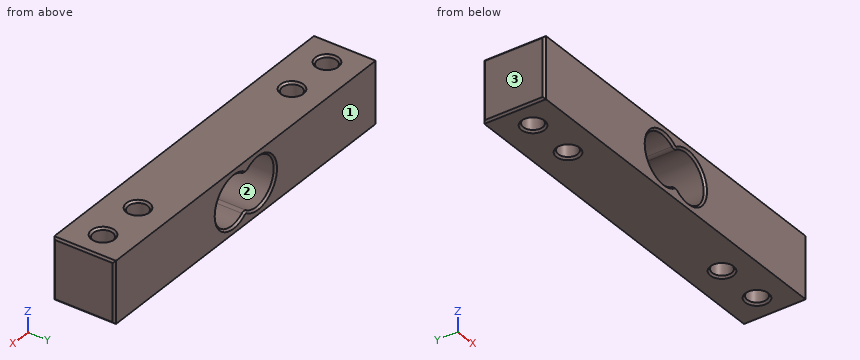
```python
from build123d import *

# Parameters (mm, degrees)
SKETCH1_W           = 75
SKETCH1_H           = 12.7
SKETCH1_R           = 2
BOSS_EXTRUDE1_DEPTH = 12.7
CUT_EXTRUDE1_REACH  = 14.7
FILLET1_R           = 1
CHAMFER1_SIZE       = 0.4


with BuildPart() as part:
    # Sketch1 → Boss-Extrude1 (new body)
    with BuildSketch(Plane.XY):
        Rectangle(SKETCH1_W, SKETCH1_H)
        with Locations((-32, 0)):
            Circle(SKETCH1_R, mode=Mode.SUBTRACT)
        with Locations((-22, 0)):
            Circle(SKETCH1_R, mode=Mode.SUBTRACT)
        with Locations((22, 0)):
            Circle(SKETCH1_R, mode=Mode.SUBTRACT)
        with Locations((32, 0)):
            Circle(SKETCH1_R, mode=Mode.SUBTRACT)
    extrude(amount=BOSS_EXTRUDE1_DEPTH)

    # Sketch2 → Cut-Extrude1 (cut, up to next)
    with BuildSketch(Plane(origin=(0, 6.35, 0), x_dir=(1, 0, 0), z_dir=(0, 1, 0)), mode=Mode.PRIVATE) as cut_extrude1_sk1:
        with BuildLine():
            ThreePointArc((0, -2.779285786), (-8.5, -6.35), (0, -9.920714214))
            ThreePointArc((0, -9.920714214), (8.5, -6.35), (0, -2.779285786))
        make_face()
    cut_extrude1_tool1 = extrude(cut_extrude1_sk1.sketch, amount=-CUT_EXTRUDE1_REACH, mode=Mode.PRIVATE) & part.part
    add(cut_extrude1_tool1.solids().sort_by_distance((0, 6.35, 6.35))[0], mode=Mode.SUBTRACT)

    # Fillet1
    fillet1_edges = [part.edges().sort_by_distance(p)[0] for p in [
        (0, 0, 2.779285786),
        (0, 0, 9.920714214),
    ]]
    fillet(fillet1_edges, radius=FILLET1_R)

    # Chamfer1
    chamfer1_edges = [part.edges().sort_by_distance(p)[0] for p in [
        (-34, 0, 0),
        (-34, 0, 12.7),
        (-37.5, 0, 12.7),
        (-24, 0, 0),
        (-24, 0, 12.7),
        (20, 0, 0),
        (20, 0, 12.7),
        (30, 0, 0),
        (30, 0, 12.7),
        (8.5, -6.35, 6.35),
        (8.5, 6.35, 6.35),
        (-8.5, 6.35, 6.35),
        (0, 6.35, 2.476602828),
        (0, 6.35, 10.223397172),
        (-8.5, -6.35, 6.35),
        (0, -6.35, 2.476602828),
        (0, -6.35, 10.223397172),
        (37.5, 0, 12.7),
        (-37.5, 0, 0),
        (37.5, 0, 0),
        (37.5, -6.35, 6.35),
        (-37.5, -6.35, 6.35),
        (-37.5, 6.35, 6.35),
        (37.5, 6.35, 6.35),
    ]]
    chamfer(chamfer1_edges, length=CHAMFER1_SIZE)


solid = part.part
```
Verification items for the finished model (mm, model axes). Face numbers are marked on the shaded views. Give positions to 0.01 mm unless a question says otherwise; leave off trailing zeros. Order: outer loops, then holes, each group sorted by start corner. A loop starts at its lowest first (then second) coordinate and runs counter-clockwise, first axis right, second up. Notation, with made-up numbers: (-5, 34) -> (54, 34) arc R23 cw to (54, 72) -> close; hole circle Ø3 at (22.5, 10.5). An arc over 180 degrees is marked (long way). Use a Markdown table: item, result.
1) Mould release check, pull along X, two halves, no side actions. Record for the marked faces 1, 2 and 3: pulls with the +X half, pulls with the -X half, needs draft (parallel to the pull), parting line crosses it, or undercut.
Results:
| item | result |
|---|---|
| face 1 | needs draft |
| face 2 | undercut |
| face 3 | pulls with the -X half |
2) Depth check by flat-ended pin: pin 1 Ø4.5 at (x, y) = (22, 0) entering from -Z; pin 2 Ø4.5 at (x, y) = (-22, 0) entering from +Z. Enter the tip coordinate at first touch or a pass-through.
Results:
| item | result |
|---|---|
| pin 1 | z = 0.15 |
| pin 2 | z = 12.55 |
3) Material ranges on probe 1 along X at (y, z) = (1.25, 6.35); probe 2 along X at (y, z) = (-3.5, 6.25); probe 3 along X at (y, z) = (0.5, 4.75), recorded low to high.
Results:
| item | result |
|---|---|
| probe 1 | -37.5 to -33.56, -30.44 to -23.56, -20.44 to -8.5, 8.5 to 20.44, 23.56 to 30.44, 33.56 to 37.5 |
| probe 2 | -37.5 to -8.5, 8.5 to 37.5 |
| probe 3 | -37.5 to -33.94, -30.06 to -23.94, -20.06 to -8.24, 8.24 to 20.06, 23.94 to 30.06, 33.94 to 37.5 |
4) Section check B-B, the plane x = -32. Record the boundary of the cut face in (y, z).
Results:
| item | result |
|---|---|
| outline | (-6.35, 0) -> (-2.4, 0) -> (-2, 0.4) -> (-2, 12.3) -> (-2.4, 12.7) -> (-6.35, 12.7) -> close; (2, 0.4) -> (2.4, 0) -> (6.35, 0) -> (6.35, 12.7) -> (2.4, 12.7) -> (2, 12.3) -> close |
5) Section check A-A, the plane z = 6.35. Record the boundary of the cut face in (x, y), then the cut area to 3 significant figures.
Results:
| item | result |
|---|---|
| outline | (-37.5, -5.95) -> (-37.1, -6.35) -> (-8.9, -6.35) -> (-8.5, -5.95) -> (-8.5, 5.95) -> (-8.9, 6.35) -> (-37.1, 6.35) -> (-37.5, 5.95) -> close; (8.5, -5.95) -> (8.9, -6.35) -> (37.1, -6.35) -> (37.5, -5.95) -> (37.5, 5.95) -> (37.1, 6.35) -> (8.9, 6.35) -> (8.5, 5.95) -> close; hole circle Ø4 at (-32, 0); hole circle Ø4 at (-22, 0); hole circle Ø4 at (22, 0); hole circle Ø4 at (32, 0) |
| area | 686 mm² |
6) Section check D-D, the plane y = -1. Give the number of separate pieces and of enclosed holes in the cut face, then the cut area to 3 significant figures.
Results:
| item | result |
|---|---|
| separate pieces | 5 |
| enclosed holes | 1 |
| area | 632 mm² |
7) Section check C-C, the plane x = 3.5. Record the boundary of the cut face in (y, z), then the cut area to 3 significant figures.
Results:
| item | result |
|---|---|
| outline | (-6.35, 0) -> (6.35, 0) -> (6.35, 0.95) -> (5.95, 1.35) -> (-5.95, 1.35) -> (-6.35, 0.95) -> close; (-6.35, 11.75) -> (-5.95, 11.35) -> (5.95, 11.35) -> (6.35, 11.75) -> (6.35, 12.7) -> (-6.35, 12.7) -> close |
| area | 34.0 mm² |
